Design review of the part built by this model. Coordinates are the model's own, in mm. Round coordinates to 2 decimals unless told otherwise and drop trailing zeros. Loops run counter-clockwise (first coordinate to the right, second up) from the corner with the lowest first, then second, coordinate; pieces in that order, holes last. Notation, with made-up numbers: (-30, 71) - (9, 71) arc R22 ccw to (9, 99) - close; hole circle Ø11 at (54, -33.5). An arc over 180 degrees is marked (long way). Use one line per item in the form item = value. Start each with the question number.
(1) We need section A-A, the plane z = 2.5. Write out the cut boundary in (x, y).
(2) Wall thickness on probe 1 along Y at (x, z) = (10, 1.5); probe 2 along Y at (x, z) = (9.5, 0.75); probe 3 along Y at (x, z) = (11.75, 3.25): over which ranges is each line inside the solid? List them lowest first. Write a range as [from, to].
(3) We need section B-B, the plane x = 10. Write out the cut boundary in (y, z), then the cut area to 3 significant figures.
(4) For pin 1 (2.5 mm diameter, centred on x = -10, y = -10, fed in from -Z), flat-tipped, find the tip position at first contact; note if it passes through.
(5) The part is to be moulded in two halves that separate along X. For faces 1 (the cylindrical face through (11.64, 11.6, 3.55)), 2 (the flat face through (0, 12.5, 3)), 3 (the cylindrical face through (8.8, -9.1, 3.5)), 4 (the cylindrical face through (-11.2, 10.9, 3.5)), say which applies: released by +X, released by -X, zero draft, split by the parting line, or undercut.
Autodesk Inventor part; units mm, degrees
ref_plane "YZ Plane" through (0, 0, 0) normal (1, 0, 0) x (0, 1, 0)
ref_plane "XZ Plane" through (0, 0, 0) normal (0, 1, 0) x (-1, 0, 0)
ref_plane "XY Plane" through (0, 0, 0) normal (0, 0, 1) x (1, 0, 0)
sketch "スケッチ1" plane through (0, 0, 0) normal (0, 0, 1) x (1, 0, 0)
  line L0 (-12.5, 12.5) -> (12.5, 12.5)
  line L1 (12.5, 12.5) -> (12.5, -12.5)
  line L2 (12.5, -12.5) -> (-12.5, -12.5)
  line L3 (-12.5, -12.5) -> (-12.5, 12.5)
  line L4 (-12.5, 12.5) -> (12.5, -12.5) construction
  line L5 (12.5, 12.5) -> (-12.5, -12.5) construction
  line L6 (10, 10) -> (-10, 10) construction
  line L7 (-10, 10) -> (-10, -10) construction
  line L8 (-10, -10) -> (10, -10) construction
  line L9 (10, -10) -> (10, 10) construction
  line L10 (10, 10) -> (-10, -10) construction
  line L11 (-10, 10) -> (10, -10) construction
  circle A0 centre (-10, 10) radius 1.5
  circle A1 centre (10, 10) radius 1.5
  circle A2 centre (-10, -10) radius 1.5
  circle A3 centre (10, -10) radius 1.5
  point P0 (0, 0)
  dimension "d0" = 25
  dimension "d1" = 25
  dimension "d2" = 20
  dimension "d3" = 20
  dimension "d4" = 3
  dimension "d5" = 3
  dimension "d6" = 3
  dimension "d7" = 3
extrude "押し出し1" add sketch "スケッチ1" along normal blind 7
fillet "フィレット1" radius 3 4 edges at (-12.5, 12.5, 3.5) (12.5, 12.5, 3.5) (12.5, -12.5, 3.5) (-12.5, -12.5, 3.5)
properties part number "YDM2507C12F"
Data:
q1.outline = (-12.5, -9.5) arc R3 ccw to (-9.5, -12.5) - (9.5, -12.5) arc R3 ccw to (12.5, -9.5) - (12.5, 9.5) arc R3 ccw to (9.5, 12.5) - (-9.5, 12.5) arc R3 ccw to (-12.5, 9.5) - close; hole circle Ø3 at (-10, -10); hole circle Ø3 at (-10, 10); hole circle Ø3 at (10, -10); hole circle Ø3 at (10, 10)
q2.probe_1 = [-12.46, -11.5], [-8.5, 8.5], [11.5, 12.46]
q2.probe_2 = [-12.5, -11.41], [-8.59, 8.59], [11.41, 12.5]
q2.probe_3 = [-11.48, 11.48]
q3.outline = (-12.46, 0) - (-11.5, 0) - (-11.5, 7) - (-12.46, 7) - close; (-8.5, 0) - (8.5, 0) - (8.5, 7) - (-8.5, 7) - close; (11.5, 0) - (12.46, 0) - (12.46, 7) - (11.5, 7) - close
q3.area = 132 mm^2
q4.pin_1 = through
q5.face_1 = released by +X
q5.face_2 = zero draft
q5.face_3 = undercut
q5.face_4 = undercut
